The figure shows three views and two pictorial views of one solid part (mm, origin at its lowest corner). Answer the questions. A direction names the side the tool comes from. Round coordinates to 2 decimals unless told otherwise and drop trailing zeros. Loops run counter-clockwise (first coordinate to the right, second up) from the corner with the lowest first, then second, coordinate; pieces in that order, holes last. Notation, with made-up numbers: (41, 23) -> (90, 23) arc R27 cw to (90, 53) -> close; hole circle Ø6 at (-27.75, 55.5). An arc over 180 degrees is marked (long way). Use a Markdown table: item, result. Add a question column.
Q1. Section A-A on x = 7 is taken. Give the vertices of the cut face in (y, z).
Q2. Consider line 1 (X direction, y = 1.55, z = 14); line 2 (Z direction, x = 27.5, y = 1.2); line 3 (Z direction, x = 7, y = 3.5). Determine where each line is inside the solid, lowest interval first.
Q3. Section B-B on z = 14 is taken. Give the vertices of the cut face in (x, y), then the cut area to 3 significant figures.
Q4. Section D-D on z = 2 is taken. Give the vertices of the cut face in (x, y).
Q5. Which of the six approach directions +Z, -Z, +X, -X, +Y, -Y give full straight-line access (tool end or side, diameter ignored) to the marked faces 1 and 2?
Q6. For a pull along Z with two mould halves and no side action, classify the marked faces 3, 4 and 5 as released by +Z, released by -Z, zero draft, split by the parting line, or undercut.
Q7. Section C-C on y = 5.25 is taken. Give the vertices of the cut face in (x, z), then the cut area to 3 significant figures.
Q8. Given pin 1 Ø10 at (x, z) = (17, 12.5) entering from +Y; pin 2 Ø4 at (y, z) = (4.5, 8) entering from +X, each flat-ended and moving along its own axis, determine where each tip first touches the part or whether it passes through.
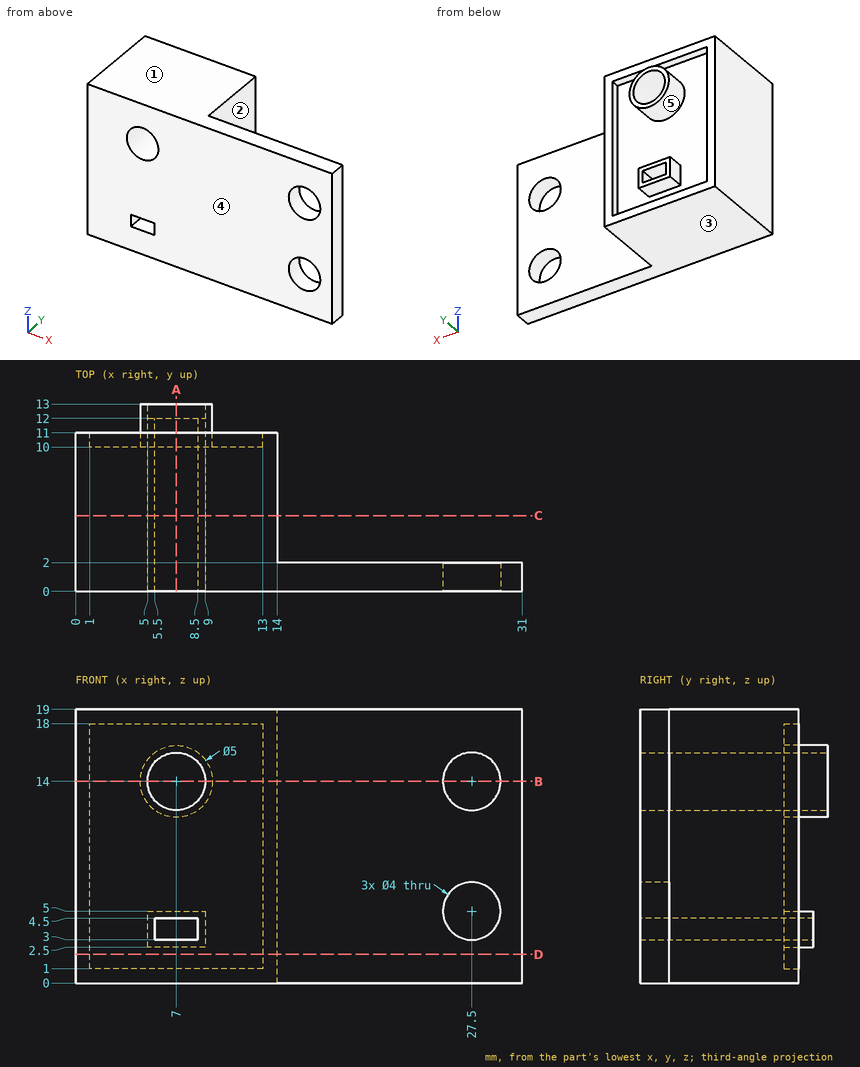
Checked values:
| question | item | result |
|---|---|---|
| 1 | outline | (0, 0) -> (11, 0) -> (11, 1) -> (10, 1) -> (10, 2.5) -> (12, 2.5) -> (12, 3) -> (0, 3) -> close; (0, 4.5) -> (12, 4.5) -> (12, 5) -> (10, 5) -> (10, 11.5) -> (13, 11.5) -> (13, 12) -> (0, 12) -> close; (0, 16) -> (13, 16) -> (13, 16.5) -> (10, 16.5) -> (10, 18) -> (11, 18) -> (11, 19) -> (0, 19) -> close |
| 2 | line 1 | x = 0 to 5, 9 to 25.5, 29.5 to 31 |
| 2 | line 2 | z = 0 to 3, 7 to 12, 16 to 19 |
| 2 | line 3 | z = 0 to 3, 4.5 to 12, 16 to 19 |
| 3 | outline | (0, 0) -> (5, 0) -> (5, 13) -> (4.5, 13) -> (4.5, 10) -> (1, 10) -> (1, 11) -> (0, 11) -> close; (9, 0) -> (25.5, 0) -> (25.5, 2) -> (14, 2) -> (14, 11) -> (13, 11) -> (13, 10) -> (9.5, 10) -> (9.5, 13) -> (9, 13) -> close; (29.5, 0) -> (31, 0) -> (31, 2) -> (29.5, 2) -> close |
| 3 | area | 131 mm2 |
| 4 | outline | (0, 0) -> (31, 0) -> (31, 2) -> (14, 2) -> (14, 11) -> (13, 11) -> (13, 10) -> (1, 10) -> (1, 11) -> (0, 11) -> close |
| 5 | face 1 | +Z, +X, -X, +Y, -Y |
| 5 | face 2 | +Z, -Z, +X, +Y |
| 6 | face 3 | released by -Z |
| 6 | face 4 | zero draft |
| 6 | face 5 | undercut |
| 7 | outline | (0, 0) -> (14, 0) -> (14, 19) -> (0, 19) -> close; hole circle Ø4 at (7, 14); hole (5.5, 3) -> (8.5, 3) -> (8.5, 4.5) -> (5.5, 4.5) -> close |
| 7 | area | 249 mm2 |
| 8 | pin 1 | stops at y = 11 |
| 8 | pin 2 | stops at x = 14 |
